Autodesk Inventor part; units mm, degrees
ref_plane "YZ Plane" through (0, 0, 0) normal (1, 0, 0) x (0, 1, 0)
ref_plane "XZ Plane" through (0, 0, 0) normal (0, 1, 0) x (-1, 0, 0)
ref_plane "XY Plane" through (0, 0, 0) normal (0, 0, 1) x (1, 0, 0)
sketch "Sketch3" plane through (0, 0, 0) normal (0, 1, 0) x (-1, 0, 0)
  line L0 (6, 6) -> (-6, 6)
  line L1 (-6, 6) -> (-6, -6)
  line L2 (-6, -6) -> (6, -6)
  line L3 (6, -6) -> (6, 6)
  line L4 (6, 6) -> (-6, -6) construction
  line L5 (-6, 6) -> (6, -6) construction
  point P0 (0, 0)
  dimension "d7" = 12
  dimension "d8" = 12
extrude "Extrusion3" add sketch "Sketch3" along normal blind 3
sketch "Sketch4" plane through (0, 3, 0) normal (0, 1, 0) x (1, 0, 0)
  circle A0 centre (0, 0) radius 3.3
  dimension "d11" = 6.6
extrude "Extrusion4" add sketch "Sketch4" along normal blind 3.2
sketch "Sketch5" plane through (0, 6.2, 0) normal (0, 1, 0) x (1, 0, 0)
  circle A0 centre (0, 0) radius 6.5
  dimension "d14" = 13
extrude "Extrusion5" add sketch "Sketch5" along normal blind 1.5
sketch "Sketch6" plane through (0, 7.7, 0) normal (0, 1, 0) x (1, 0, 0)
  circle A0 centre (0, 0) radius 5.75
  dimension "d17" = 11.5
extrude "Extrusion6" add sketch "Sketch6" along normal blind 4.1
sketch "Sketch7" plane through (-6, 0, -6) normal (-1, 0, 0) x (0, 0, 1)
  line L0 (3, -0.4) -> (9, -0.4)
  line L1 (9, -0.4) -> (9, 0.4)
  line L2 (9, 0.4) -> (3, 0.4)
  line L3 (3, 0.4) -> (3, -0.4)
  line L4 (3, -0.4) -> (9, 0.4) construction
  line L5 (9, -0.4) -> (3, 0.4) construction
  line L6 (4, -0.4) -> (8, -0.4)
  line L7 (8, -0.4) -> (8, 0.4)
  line L8 (8, 0.4) -> (4, 0.4)
  line L9 (4, 0.4) -> (4, -0.4)
  line L10 (4, -0.4) -> (8, 0.4) construction
  line L11 (8, -0.4) -> (4, 0.4) construction
  line L12 (0, 0) -> (12, 0)
  point P0 (6, 0)
  point P1 (8, 0)
  point P2 (9, 0)
  point P3 (3, 0)
  point P4 (4, 0)
  dimension "d20" = 6
  dimension "d21" = 0.8
  dimension "d22" = 4
extrude "Extrusion7" add sketch "Sketch7" along normal blind 4 contours L3 L2 L9 L12 | L7 L2 L1 L12
mirror "Mirror1" about plane through (0, 0, 0) normal (1, 0, 0) of "Extrusion7"
properties part number "Button"
Part model, mm, in its own coordinate system. A direction names the side the tool comes from. Coordinates: 2 decimals unless noted, no trailing zeros. Order: outer loops, then holes, each group sorted by start corner. A loop starts at its lowest first (then second) coordinate and runs counter-clockwise, first axis right, second up. Notation, with made-up numbers: (-25, 31) - (27, 31) arc R32 cw to (27, 66) - close; hole circle Ø7 at (87, 49.5). An arc over 180 degrees is marked (long way). Return JSON: item names as keys, results as strings. Group by question number.
Item 1: Pin check, flat tips, straight feed: pin 1 (1 mm diameter, centred on y = 3, z = -0.5, fed in from +X); pin 2 (5 mm diameter, centred on y = 4.5, z = 2, fed in from +X); pin 3 (0.8 mm diameter, centred on x = 7.5, z = -2.5, fed in from +Y); pin 4 (6.5 mm diameter, centred on x = 1, z = 0.5, fed in from -Y). Stop position of each tip, or through.
Item 2: Drill centre lines: probe 1 along Y at (x, z) = (3.25, 5.5); probe 2 along Y at (x, z) = (5, 2.5); probe 3 along Z at (x, y) = (-1, 2.25). Where is each one in solid material? Low to high. Write a range as from..to.
Item 3: Which spindle directions (+Z, -Z, +X, -X, +Y, -Y) get a long thin tool onto all of the face, cutting with end or side? Do faces 1 (the face through (0, 1, -6)), 2 (the face through (-5.158, 6.94, -3.955)), 3 (the face through (0, 1, 6)), 4 (the face through (-3, 3, 3)). Say none if no direction does.
Item 4: Cut at C-C (z = 0). List the corners of the cut face in (x, y), plus the area to 3 significant figures.
Item 5: Pull direction Y, two halves, no side cores. Call faces 5 (the face through (-0.75, 9.72, 5.7)), 6 (the face through (-2.43, 4.58, 2.23)), 7 (the face through (0, 0, 0)): pulls with the +Y half, pulls with the -Y half, needs draft (parallel to the pull), parting line crosses it, or undercut.
Item 6: Cut at A-A (x = -7). List the corners of the cut face in (y, z), plus the area to 3 significant figures.
Item 7: Cut at D-D (x = 1.75). List the corners of the cut face in (y, z), plus the area to 3 significant figures.
Item 8: Cut at B-B (z = 4.75). List the corners of the cut face in (x, y).
Check values:
{
 "1": {"pin 1": "stops at x = 6", "pin 2": "stops at x = 6.5", "pin 3": "stops at y = 0.4", "pin 4": "stops at y = 0"},
 "2": {"probe 1": "y = 0..3, 6.2..7.7", "probe 2": "y = 0..3, 6.2..11.8", "probe 3": "z = -6..6"},
 "3": {"face 1": "-Z, +X, -X, -Y", "face 2": "+Y", "face 3": "+Z, +X, -X, -Y", "face 4": "none"},
 "4": {"outline": "(-6.5, 6.2) - (-3.3, 6.2) - (-3.3, 3) - (-6, 3) - (-6, 0) - (6, 0) - (6, 3) - (3.3, 3) - (3.3, 6.2) - (6.5, 6.2) - (6.5, 7.7) - (5.75, 7.7) - (5.75, 11.8) - (-5.75, 11.8) - (-5.75, 7.7) - (-6.5, 7.7) - close", "area": "124 mm2"},
 "5": {"face 5": "needs draft", "face 6": "undercut", "face 7": "pulls with the -Y half"},
 "6": {"outline": "(0, -3) - (0.4, -3) - (0.4, -2) - (0, -2) - close; (0, 2) - (0.4, 2) - (0.4, 3) - (0, 3) - close", "area": "0.800 mm2"},
 "7": {"outline": "(0, -6) - (3, -6) - (3, -2.8) - (6.2, -2.8) - (6.2, -6.26) - (7.7, -6.26) - (7.7, -5.48) - (11.8, -5.48) - (11.8, 5.48) - (7.7, 5.48) - (7.7, 6.26) - (6.2, 6.26) - (6.2, 2.8) - (3, 2.8) - (3, 6) - (0, 6) - close", "area": "118 mm2"},
 "8": {"outline": "(-6, 0) - (6, 0) - (6, 3) - (-6, 3) - close; (-4.44, 6.2) - (4.44, 6.2) - (4.44, 7.7) - (3.24, 7.7) - (3.24, 11.8) - (-3.24, 11.8) - (-3.24, 7.7) - (-4.44, 7.7) - close"}
}
